```python
from build123d import *

# Parameters (mm, degrees)
SKETCH1_W      = 65
SKETCH1_H      = 58
EXTRUDE1_DEPTH = 9.5
EXTRUDE2_DEPTH = 66
EXTRUDE3_DEPTH = 66
SKETCH4_W      = 30
SKETCH4_H      = 18.1
EXTRUDE4_DEPTH = 65
SKETCH5_R      = 2.1
EXTRUDE5_DEPTH = 28.6
SKETCH6_R      = 4
EXTRUDE6_DEPTH = 20


with BuildPart() as part:
    # Sketch1 → Extrude1 (new body)
    with BuildSketch(Plane(origin=(0, 0, 0), x_dir=(1, 0, 0), z_dir=(0, 1, 0))):
        with Locations((32.5, 29)):
            Rectangle(SKETCH1_W, SKETCH1_H)
    extrude(amount=EXTRUDE1_DEPTH)

    # Sketch2 → Extrude2 (cut, through all)
    with BuildSketch(Plane(origin=(65, 0, 0), x_dir=(0, 0, -1), z_dir=(1, 0, 0))):
        Polygon((0, 0), (5.484827557, 9.5), (0, 9.5), align=None)
    extrude(amount=-EXTRUDE2_DEPTH, mode=Mode.SUBTRACT)

    # Sketch3 → Extrude3 (cut, through all)
    with BuildSketch(Plane(origin=(65, 0, 0), x_dir=(0, 0, -1), z_dir=(1, 0, 0))):
        Polygon((58, 0), (58, 4.7), (55.8, 3.176135582), align=None)
    extrude(amount=-EXTRUDE3_DEPTH, mode=Mode.SUBTRACT)

    # Sketch4 → Extrude4 (add)
    with BuildSketch(Plane.ZY):
        with Locations((-31, 18.55)):
            Rectangle(SKETCH4_W, SKETCH4_H)
    extrude(amount=-EXTRUDE4_DEPTH)

    # Sketch5 → Extrude5 (cut, through all)
    with BuildSketch(Plane(origin=(0, 27.6, 0), x_dir=(1, 0, 0), z_dir=(0, 1, 0))):
        with Locations(Location((50, 31, 0), (0, 0, 270))):  # turned: the seam where the file's is
            Circle(SKETCH5_R)
    extrude(amount=-EXTRUDE5_DEPTH, mode=Mode.SUBTRACT)

    # Sketch6 → Extrude6 (cut)
    with BuildSketch(Plane.XZ):
        with Locations(Location((50, -31, 0), (0, 0, 270))):  # turned: the seam where the file's is
            Circle(SKETCH6_R)
    extrude(amount=-EXTRUDE6_DEPTH, mode=Mode.SUBTRACT)


solid = part.part
```
Check sheet for the modelled part. Datum: model origin and axes. Units: mm. A direction names the side the tool comes from. Coordinates: 2 decimals unless noted, no trailing zeros. Loops run counter-clockwise (first coordinate to the right, second up) from the corner with the lowest first, then second, coordinate; pieces in that order, holes last.
1) Sectioned sample at C-C (y = 21.5). Record the boundary of the cut face in (x, z).
2) Sectioned sample at D-D (x = 32.5). Record the boundary of the cut face in (y, z).
3) Sectioned sample at B-B (x = 50). Record the boundary of the cut face in (y, z), and give its area (3 significant figures).
4) Material ranges on probe 1 along X at (y, z) = (13.75, -31); probe 2 along X at (y, z) = (25.25, -31); probe 3 along Z at (x, y) = (35.5, 26), recorded low to high.
5) Sectioned sample at A-A (z = -31). Record the boundary of the cut face in (x, y), and give its area (3 significant figures).
6) Release check for a two-part mould opening along Z. For faces 6 (the face through (32, 9.5, -52)), 7 (the face through (32, 18, -16)), 8 (the face through (48, 20, -33)) record: released by +Z, released by -Z, zero draft, split by the parting line, or undercut.
7) Gauge pin test, flat ends, axial feed: pin 1 (8 mm diameter, centred on x = 17, y = 22.5, fed in from -Z); pin 2 (10 mm diameter, centred on x = 15.5, y = 15.5, fed in from +Z); pin 3 (5.5 mm diameter, centred on x = 26, z = -10, fed in from +Y); pin 4 (6 mm diameter, centred on x = 13.5, z = -25.5, fed in from -Y). Record the tip position at first contact, or that the pin passes through.
8) Access from +Z, -Z, +X, -X, +Y, -Y to the whole of each face (thin tool, end or side, straight path). Record for faces 1 (the face through (32, 18, -46)), 2 (the face through (32.955, 1.61, -56.885)), 3 (the face through (32, 0, -29)), 4 (the face through (46.451, 9.86, -32.846)), 5 (the face through (32, 9.5, -11)).
Check sheet entries:
1. outline: (0, -46) - (65, -46) - (65, -16) - (0, -16) - close; hole circle Ø4.2 at (50, -31)
2. outline: (0, -58) - (3.18, -55.8) - (4.7, -58) - (9.5, -58) - (9.5, -46) - (27.6, -46) - (27.6, -16) - (9.5, -16) - (9.5, -5.48) - (0, 0) - close
3. outline: (0, -58) - (3.18, -55.8) - (4.7, -58) - (9.5, -58) - (9.5, -46) - (27.6, -46) - (27.6, -33.1) - (20, -33.1) - (20, -35) - (0, -35) - close; (0, -27) - (20, -27) - (20, -28.9) - (27.6, -28.9) - (27.6, -16) - (9.5, -16) - (9.5, -5.48) - (0, 0) - close
3. area: 871 mm2
4. probe 1: x = 0 to 46, 54 to 65
4. probe 2: x = 0 to 47.9, 52.1 to 65
4. probe 3: z = -46 to -16
5. outline: (0, 0) - (46, 0) - (46, 20) - (47.9, 20) - (47.9, 27.6) - (0, 27.6) - close; (52.1, 20) - (54, 20) - (54, 0) - (65, 0) - (65, 27.6) - (52.1, 27.6) - close
5. area: 1,600 mm2
6. face 6: zero draft
6. face 7: released by +Z
6. face 8: undercut
7. pin 1: stops at z = -46
7. pin 2: stops at z = -16
7. pin 3: stops at y = 9.5
7. pin 4: stops at y = 0
8. face 1: -Z, +X, -X, +Y
8. face 2: -Z, +X, -X
8. face 3: +Z, -Z, +X, -X, -Y
8. face 4: -Y
8. face 5: +Z, +X, -X, +Y
